Geometry: final body of the model. Coordinates: model frame, mm. Coordinates: 2 decimals unless noted, no trailing zeros. Loops run counter-clockwise (first coordinate to the right, second up) from the corner with the lowest first, then second, coordinate; pieces in that order, holes last. Notation, with made-up numbers: (38.25, -8) - (53.25, -8) arc R25 cw to (53.25, 12) - close; hole circle Ø1 at (65.5, -1.75). An arc over 180 degrees is marked (long way). Answer in a Markdown table with one row per item.
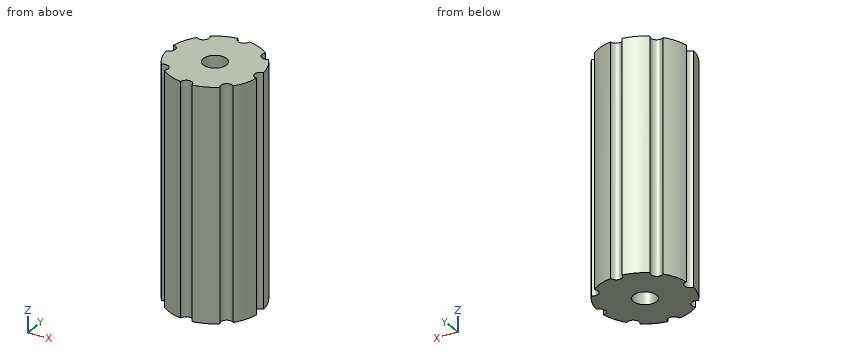
Solid Edge part; units mm, degrees
sketch "Sketch1" plane through (0, 0, 0) normal (0, 0, 1) x (1, 0, 0)
  arc A0 (3.9688, -0.499) -> (3.1592, -2.4535) centre (0, 0) cw
  arc A1 (2.4535, -3.1592) -> (0.499, -3.9688) centre (0, 0) cw
  arc A2 (-0.499, -3.9688) -> (-2.4535, -3.1592) centre (0, 0) cw
  arc A3 (-3.1592, -2.4535) -> (-3.9688, -0.499) centre (0, 0) cw
  arc A4 (-3.9688, 0.499) -> (-3.1592, 2.4535) centre (0, 0) cw
  arc A5 (-2.4535, 3.1592) -> (-0.499, 3.9688) centre (0, 0) cw
  arc A6 (0.499, 3.9688) -> (2.4535, 3.1592) centre (0, 0) cw
  arc A7 (2.4535, -3.1592) -> (3.1592, -2.4535) centre (2.8284, -2.8284) cw
  arc A8 (-0.499, -3.9688) -> (0.499, -3.9688) centre (0, -4) cw
  arc A9 (-3.1592, -2.4535) -> (-2.4535, -3.1592) centre (-2.8284, -2.8284) cw
  arc A10 (-3.9688, 0.499) -> (-3.9688, -0.499) centre (-4, 0) cw
  arc A11 (-2.4535, 3.1592) -> (-3.1592, 2.4535) centre (-2.8284, 2.8284) cw
  arc A12 (0.499, 3.9688) -> (-0.499, 3.9688) centre (0, 4) cw
  arc A13 (3.1592, 2.4535) -> (2.4535, 3.1592) centre (2.8284, 2.8284) cw
  arc A14 (3.1592, 2.4535) -> (3.9688, 0.499) centre (0, 0) cw
  arc A15 (3.9688, -0.499) -> (3.9688, 0.499) centre (4, 0) cw
  circle A16 centre (0, 0) radius 1
extrude "Protrusion1" add sketch "Sketch1" along normal blind 20
(1) Cut plane A-A on y = 0. Output: boundary loops of the cut face in (x, z).
Verdict:
| item | result |
|---|---|
| outline | (-3.5, 0) - (-1, 0) - (-1, 20) - (-3.5, 20) - close; (1, 0) - (3.5, 0) - (3.5, 20) - (1, 20) - close |
(2) First-contact query: pin 1 Ø1 at (x, z) = (-1.5, 15.5) entering from -Y; pin 2 Ø1.2 at (x, y) = (0, 0) entering from +Z; pin 3 Ø4 at (x, z) = (-2.5, 9) entering from +Y. Flat tips, straight axial feed; report the tip coordinate or a pass-through.
Verdict:
| item | result |
|---|---|
| pin 1 | stops at y = -3.87 |
| pin 2 | passes through |
| pin 3 | stops at y = 3.97 |
(3) Ray query, probe 1 along Y at (x, z) = (0, 8); probe 2 along X at (y, z) = (-0.25, 8); probe 3 along Y at (x, z) = (0.75, 13.5). Return the intervals inside material, ascending.
Verdict:
| item | result |
|---|---|
| probe 1 | y = -3.5 to -1, 1 to 3.5 |
| probe 2 | x = -3.57 to -0.97, 0.97 to 3.57 |
| probe 3 | y = -3.93 to -0.66, 0.66 to 3.93 |
(4) Cut plane C-C on z = 7. Output: boundary loops of the cut face in (x, y), then the cut area to 3 significant figures.
Verdict:
| item | result |
|---|---|
| outline | (-3.97, -0.5) arc R4 ccw to (-3.16, -2.45) arc R0.5 cw to (-2.45, -3.16) arc R4 ccw to (-0.5, -3.97) arc R0.5 cw to (0.5, -3.97) arc R4 ccw to (2.45, -3.16) arc R0.5 cw to (3.16, -2.45) arc R4 ccw to (3.97, -0.5) arc R0.5 cw to (3.97, 0.5) arc R4 ccw to (3.16, 2.45) arc R0.5 cw to (2.45, 3.16) arc R4 ccw to (0.5, 3.97) arc R0.5 cw to (-0.5, 3.97) arc R4 ccw to (-2.45, 3.16) arc R0.5 cw to (-3.16, 2.45) arc R4 ccw to (-3.97, 0.5) arc R0.5 cw to start; hole circle Ø2 at (0, 0) |
| area | 44.1 mm² |
(5) Cut plane D-D on y = -2. Output: boundary loops of the cut face in (x, z).
Verdict:
| item | result |
|---|---|
| outline | (-3.46, 0) - (3.46, 0) - (3.46, 20) - (-3.46, 20) - close |
